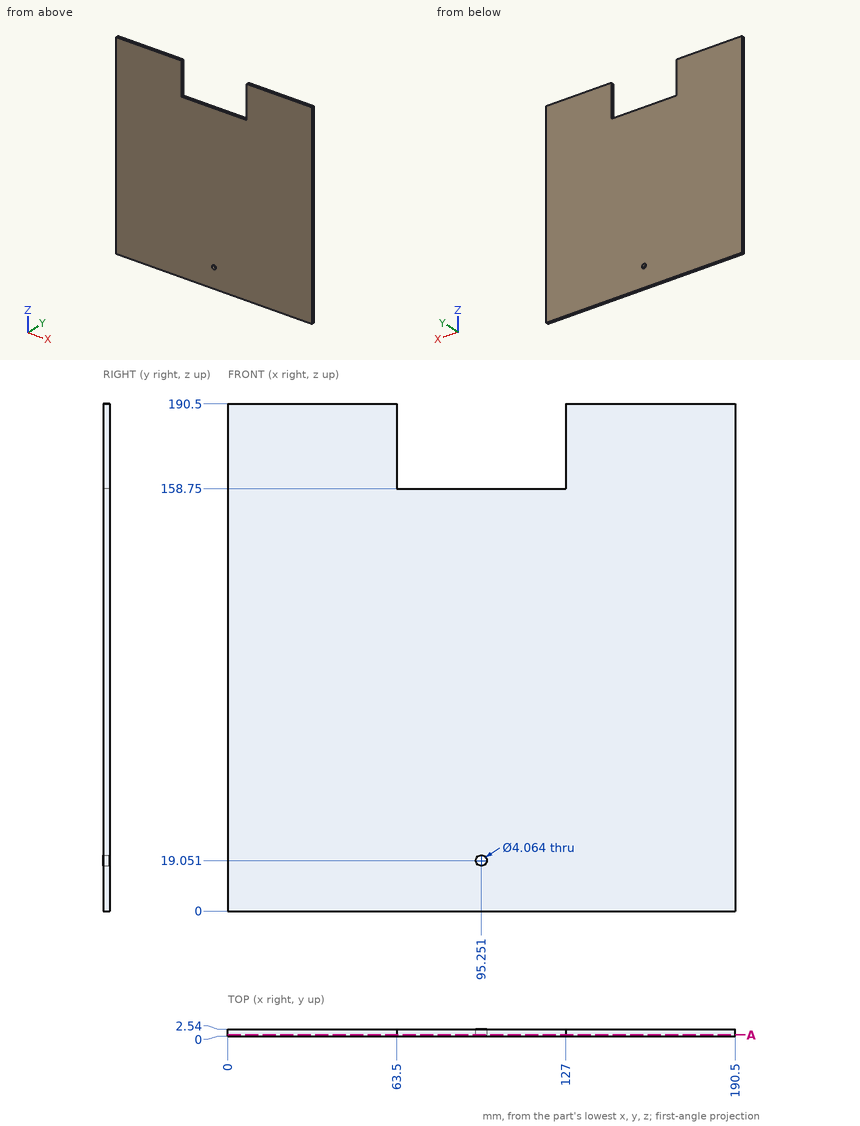
Geometry: see drawing. Coordinates: mm, zero at the bounding-box minimum. Round coordinates to 2 decimals unless told otherwise and drop trailing zeros. Write each loop counter-clockwise with the first axis right and the second up, starting at its lowest first coordinate (ties: lowest second). Pieces come first, ordered by that corner, then holes.
Item 1: Material intervals for L1, parallel to X at y = 2.35, z = 179; L2, parallel to Z at x = 83, y = 2.2; L3, parallel to Z at x = 94, y = 1.25, sorted ascending.
Item 2: Section query A-A (y = 0.45). Return loops of the section in (x, z).
Item 3: Pin query (flat end, axial travel): P1, Ø1.3, axis at x = 102, y = 1, coming from the +Z side. Return the tip coordinate at first contact, or that it passes through.
Completed:
1. L1: x = 0 to 63.5, 127 to 190.5
1. L2: z = 0 to 158.75
1. L3: z = 0 to 17.45, 20.65 to 158.75
2. outline: (0, 0) - (190.5, 0) - (190.5, 190.5) - (127, 190.5) - (127, 158.75) - (63.5, 158.75) - (63.5, 190.5) - (0, 190.5) - close; hole circle Ø4.06 at (95.25, 19.05)
3. P1: stops at z = 158.75
